from build123d import *

# Parameters (mm, degrees)
SKETCH_W        = 29
SKETCH_H        = 54
PAD_DEPTH       = 4
SKETCH001_W     = 15
SKETCH001_H     = 40
POCKET_DEPTH    = 5
SKETCH002_R     = 2
POCKET001_DEPTH = 4.001
SKETCH003_W     = 25
SKETCH003_H     = 20
PAD001_DEPTH    = 10
SKETCH004_R     = 2
POCKET002_DEPTH = 14.001
SKETCH006_W     = 8
SKETCH006_H     = 3
POCKET003_DEPTH = 17
CHAMFER_SIZE    = 3.9


with BuildPart() as part:
    # Sketch → Pad (new body)
    with BuildSketch(Plane.XZ):
        Rectangle(SKETCH_W, SKETCH_H)
    extrude(amount=PAD_DEPTH)

    # Sketch001 (on Face6 of Pad) → Pocket (cut)
    with BuildSketch(Plane.XZ.offset(4)):
        Rectangle(SKETCH001_W, SKETCH001_H)
    extrude(amount=-POCKET_DEPTH, mode=Mode.SUBTRACT)

    # Sketch002 (on Face5 of Pocket) → Pocket001 (cut, through all)
    with BuildSketch(Plane.XZ.offset(4)):
        with Locations((-5, 23.5)):
            Circle(SKETCH002_R)
        with Locations((5, 23.5)):
            Circle(SKETCH002_R)
        with Locations((-5, -23.5)):
            Circle(SKETCH002_R)
        with Locations((5, -23.5)):
            Circle(SKETCH002_R)
    extrude(amount=-POCKET001_DEPTH, mode=Mode.SUBTRACT)

    # Sketch003 (on Face5 of Pocket001) → Pad001 (join)
    with BuildSketch(Plane.XZ.offset(4)):
        with Locations((0.25, -10)):
            Rectangle(SKETCH003_W, SKETCH003_H)
    extrude(amount=PAD001_DEPTH)

    # Sketch004 (on Face20 of Pad001) → Pocket002 (cut, through all)
    with BuildSketch(Plane.XZ.offset(14)):
        with Locations((0, -6)):
            Circle(SKETCH004_R)
        with Locations((0, -15)):
            Circle(SKETCH004_R)
    extrude(amount=-POCKET002_DEPTH, mode=Mode.SUBTRACT)

    # Sketch006 (on Face16 of Pocket002) → Pocket003 (cut)
    with BuildSketch(Plane(origin=(12.75, 0, 0), x_dir=(0, 0, 1), z_dir=(1, 0, 0))):
        with Locations((-14.5, 9)):
            Rectangle(SKETCH006_W, SKETCH006_H)
        with Locations((-4.5, 9)):
            Rectangle(SKETCH006_W, SKETCH006_H)
    extrude(amount=-POCKET003_DEPTH, mode=Mode.SUBTRACT)

    # Chamfer
    chamfer_edges = [part.edges().sort_by_distance(p)[0] for p in [
        (-4.25, -9, -18.5),
        (-4.25, -9, -0.5),
        (-4.25, -9, -8.5),
        (-4.25, -9, -10.5),
    ]]
    chamfer(chamfer_edges, length=CHAMFER_SIZE)


solid = part.part
Geometry: final body of the model. Coordinates: model frame, mm. A direction names the side the tool comes from. Round coordinates to 2 decimals unless told otherwise and drop trailing zeros. Loops run counter-clockwise (first coordinate to the right, second up) from the corner with the lowest first, then second, coordinate; pieces in that order, holes last. Notation, with made-up numbers: M 14.5,66 L 28.5,66 A35 cw 28.5,104 Z; hole C 45.25,29.5 d6. An arc over 180 degrees is marked long. Put each result on its own line as item: value. Start each with the question number.
(1) Section query D-D (y = -5.25). Return loops of the section in (x, z).
(2) Section query C-C (z = 10.5). Return loops of the section in (x, y).
(3) Material intervals for line 1 along Z through (x, y) = (1.25, -8.75); line 2 along Z through (x, y) = (5, -2.6); line 3 along Z through (x, y) = (0, -4.85), sorted ascending. Write a range as [from, to].
(4) Section query B-B (z = -23.5). Return loops of the section in (x, y), then the cut area to 3 significant figures.
(5) Set-up query: faces 4 (the face through (6, -10.5, -15)), 5 (the face through (0, -2, 20)), 6 (the face through (12.75, -9, -10)), 7 (the face through (-12.25, -9, -10)), 8 (the face through (-7.5, -2, 0)). Return all of +Z, -Z, +X, -X, +Y, -Y with unobstructed straight access to the full face (end or side cutting, diameter ignored); none if empty.
(6) Contact query for flat-ended pins moving along their axis: pin 1 Ø1.5 at (x, y) = (0, -11) entering from +Z; pin 2 Ø2.5 at (x, z) = (0, -15) entering from -Y; pin 3 Ø3 at (y, z) = (-9.5, -18) entering from +X; pin 4 Ø2.5 at (x, y) = (5.5, -9) entering from -Z. Output: stop coordinate, or through.
(7) Draft query along Y for faces 1 (the face through (0, -9, 0)), 2 (the face through (6, -7.5, -5)), 3 (the face through (0, -4, -10)). Return one class per face: +Y half, -Y half, draft (parallel to the pull), parting line (faces both ways), or undercut.
Findings below:
1. outline: M -12.25,-20 L 12.75,-20 L 12.75,0 L -12.25,0 Z; hole C 0,-15 d4; hole C 0,-6 d4
2. outline: M -14.5,-4 L -7.5,-4 L -7.5,0 L -14.5,0 Z; M 7.5,-4 L 14.5,-4 L 14.5,0 L 7.5,0 Z
3. line 1: z = [-20, -18.5], [-10.5, -8.5], [-0.5, 0]
3. line 2: z = [-27, -25.5], [-21.5, -20], [20, 21.5], [25.5, 27]
3. line 3: z = [-20, -17], [-13, -8], [-4, 0]
4. outline: M -14.5,-4 L -7,-4 L -7,0 L -14.5,0 Z; M -3,-4 L 3,-4 L 3,0 L -3,0 Z; M 7,-4 L 14.5,-4 L 14.5,0 L 7,0 Z
4. area: 84.0 mm2
5. face 4: +X
5. face 5: +Y, -Y
5. face 6: +Z, -Z, +X, -Y
5. face 7: +Z, -Z, -X, -Y
5. face 8: +Y
6. pin 1: stops at z = 0
6. pin 2: passes through
6. pin 3: stops at x = 12.75
6. pin 4: stops at z = -20
7. face 1: draft
7. face 2: undercut
7. face 3: +Y half
